```python
from build123d import *

# Parameters (mm, degrees)
EXTRUDE_1_OUTLINE_W = 215
EXTRUDE_1_OUTLINE_H = 235
EXTRUDE_1_DEPTH     = 5
SKETCH_3_W          = 150
SKETCH_3_H          = 55
CUT_EXTRUDE_1_DEPTH = 1813.363972104
EXTRUDE_1_2_DEPTH   = 15
SKETCH_5_W          = 55
SKETCH_5_H          = 55
CUT_EXTRUDE_2_DEPTH = 1813.419147819


# Read off the part's stored shape, not the designer's step: 凸台-拉伸1
with BuildPart() as part:
    # Extrude 1 outline → Extrude 1 (new body)
    with BuildSketch(Plane(origin=(0, 0, 0), x_dir=(1, 0, 0), z_dir=(0, 1, 0))):
        with Locations((-564.05165919, -1565.846825945)):
            Rectangle(EXTRUDE_1_OUTLINE_W, EXTRUDE_1_OUTLINE_H)
    extrude(amount=EXTRUDE_1_DEPTH)

    # 草图3 → 切除-拉伸1 (cut, through all)
    with BuildSketch(Plane(origin=(0, 5, 0), x_dir=(1, 0, 0), z_dir=(0, 1, 0))):
        with Locations((-531.55165919, -1475.846825945)):
            Rectangle(SKETCH_3_W, SKETCH_3_H)
    extrude(amount=-CUT_EXTRUDE_1_DEPTH, mode=Mode.SUBTRACT)

    # 草图4 → Extrude 1 2 (add)
    with BuildSketch(Plane(origin=(0, 5, 0), x_dir=(1, 0, 0), z_dir=(0, 1, 0))):
        Polygon((-456.55165919, -1503.346825945), (-606.55165919, -1503.346825945), (-606.55165919, -1448.346825945), (-671.55165919, -1448.346825945), (-671.55165919, -1683.346825945), (-456.55165919, -1683.346825945), align=None)
        Polygon((-461.55165919, -1508.346825945), (-611.55165919, -1508.346825945), (-611.55165919, -1453.346825945), (-666.55165919, -1453.346825945), (-666.55165919, -1678.346825945), (-461.55165919, -1678.346825945), align=None, mode=Mode.SUBTRACT)
    extrude(amount=EXTRUDE_1_2_DEPTH)

    # 草图5 → 切除-拉伸2 (cut, through all)
    with BuildSketch(Plane(origin=(0, 5, 0), x_dir=(1, 0, 0), z_dir=(0, 1, 0))):
        with Locations((-639.05165919, -1480.846825945)):
            Rectangle(SKETCH_5_W, SKETCH_5_H)
    extrude(amount=-CUT_EXTRUDE_2_DEPTH, mode=Mode.SUBTRACT)


solid = part.part
```
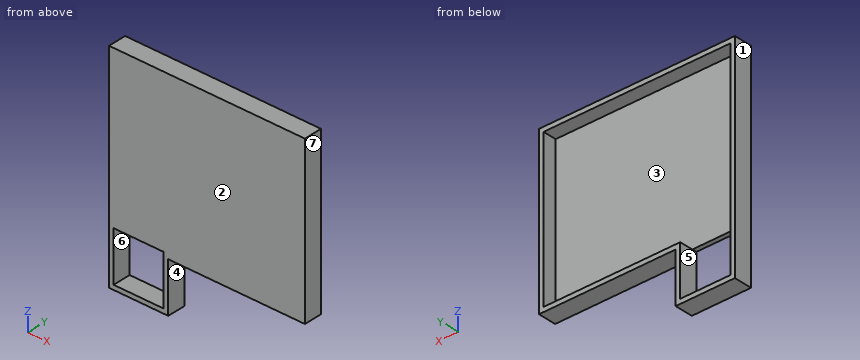
Input: part model. Units: mm. Frame: model coordinates. Face numbers are marked on the shaded views. A direction names the side the tool comes from. Coordinates: 2 decimals unless noted, no trailing zeros. Order: outer loops, then holes, each group sorted by start corner. A loop starts at its lowest first (then second) coordinate and runs counter-clockwise, first axis right, second up. Notation, with made-up numbers: (50.25, -29.75) - (57.25, -29.75) arc R27 ccw to (57.25, 0.25) - close; hole circle Ø1 at (58, -32.75). An arc over 180 degrees is marked (long way). Put each result on its own line as item: value.
1. Cut plane A-A on x = -626. Return the cut outline in (y, z), then the cut area to 3 significant figures.
Report:
outline: (0, 1448.35) - (20, 1448.35) - (20, 1453.35) - (0, 1453.35) - close; (0, 1508.35) - (5, 1508.35) - (5, 1678.35) - (20, 1678.35) - (20, 1683.35) - (0, 1683.35) - close
area: 1,050 mm2
2. Reachability of the marked faces 1, 2, 3, 4 and 5 from +Z, -Z, +X, -X, +Y, -Y: full face, straight path, thin tool, end or side. Return the list, or none.
Report:
face 1: +Z, -Z, -X, +Y, -Y
face 2: +Z, -Z, +X, -X, -Y
face 3: +Y
face 4: -Z, +X, +Y, -Y
face 5: +Y, -Y
3. Line query: line 1 along Z through (x, y) = (-470, 6.75); line 2 along Z through (x, y) = (-662.5, 2.75); line 3 along X through (y, z) = (6, 1570). Output: solid intervals per line, ascending.
Report:
line 1: z = 1503.35 to 1508.35, 1678.35 to 1683.35
line 2: z = 1448.35 to 1453.35, 1508.35 to 1683.35
line 3: x = -671.55 to -666.55, -461.55 to -456.55
4. Draft query along Z for the marked faces 6 and 7. Return one class per face: pulls with the +Z half, pulls with the -Z half, needs draft (parallel to the pull), parting line crosses it, or undercut.
Report:
face 6: undercut
face 7: needs draft
5. Cut plane B-B on y = 15.5. Return the cut outline in (x, z), then the cut area to 3 significant figures.
Report:
outline: (-671.55, 1448.35) - (-606.55, 1448.35) - (-606.55, 1503.35) - (-456.55, 1503.35) - (-456.55, 1683.35) - (-671.55, 1683.35) - close; hole (-666.55, 1453.35) - (-611.55, 1453.35) - (-611.55, 1508.35) - (-461.55, 1508.35) - (-461.55, 1678.35) - (-666.55, 1678.35) - close
area: 4,400 mm2
6. Cut plane D-D on x = -495. Return the cut outline in (y, z), then the cut area to 3 significant figures.
Report:
outline: (0, 1503.35) - (20, 1503.35) - (20, 1508.35) - (5, 1508.35) - (5, 1678.35) - (20, 1678.35) - (20, 1683.35) - (0, 1683.35) - close
area: 1,050 mm2
7. Cut plane C-C on z = 1566.5. Return the cut outline in (x, y), then the cut area to 4 significant figures.
Report:
outline: (-671.55, 0) - (-456.55, 0) - (-456.55, 20) - (-461.55, 20) - (-461.55, 5) - (-666.55, 5) - (-666.55, 20) - (-671.55, 20) - close
area: 1,225 mm2
8. Contact query for flat-ended pins moving along their axis: pin 1 Ø10 at (x, y) = (-562, 10.5) entering from -Z; pin 2 Ø6 at (x, z) = (-547.5, 1567.5) entering from +Y. Output: stop coordinate, or through.
Report:
pin 1: stops at z = 1503.35
pin 2: stops at y = 5
